from build123d import *

# Parameters (mm, degrees)
F2_ANGLE = 90
F0_W     = 20.32
F0_H     = 20.32
F3_DEPTH = 34.361461
F4_R     = 3.302
F5_DEPTH = 34.361461


with BuildPart() as f2:
    # F1 (on Right) → F2 (revolve)
    with BuildSketch(Plane.YZ):
        with BuildLine():
            ThreePointArc((44.45, -10.16), (34.29, 0), (44.45, 10.16))
            Line((44.45, 10.16), (44.45, 17.18023))
            Line((44.45, 17.18023), (0, 17.18023))
            Line((0, 17.18023), (0, 0))
            Line((0, 0), (0, -17.18023))
            Line((0, -17.18023), (44.45, -17.18023))
            Line((44.45, -17.18023), (44.45, -10.16))
        make_face()
    revolve(axis=Axis((0, 0, 26.599785), (0, 0, 1)), revolution_arc=F2_ANGLE)

    # F0 (on face) → F3 (cut, through all)
    with BuildSketch(Plane(origin=(0, 0, -17.18023), x_dir=(1, 0, 0), z_dir=(0, 0, -1))):
        with Locations((-10.16, -10.16)):
            Rectangle(F0_W, F0_H)
    extrude(amount=-F3_DEPTH, mode=Mode.SUBTRACT)

    # F4 (on face) → F5 (cut, through all)
    with BuildSketch(Plane(origin=(0, 0, -17.18023), x_dir=(1, 0, 0), z_dir=(0, 0, -1))):
        with Locations((-29.21, -7.62)):
            Circle(F4_R)
        with Locations((-7.62, -29.21)):
            Circle(F4_R)
    extrude(amount=-F5_DEPTH, mode=Mode.SUBTRACT)


solid = f2.part
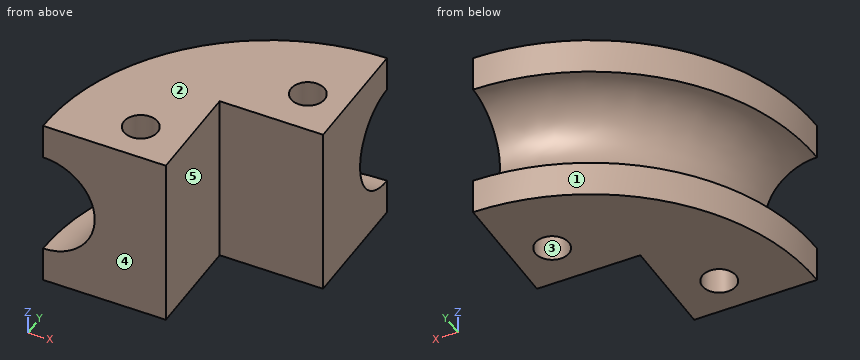
The model under review builds one solid part; all positions refer to its coordinate system, in mm. Face numbers are marked on the shaded views. A direction names the side the tool comes from. Coordinates: 2 decimals unless noted, no trailing zeros. Order: outer loops, then holes, each group sorted by start corner. A loop starts at its lowest first (then second) coordinate and runs counter-clockwise, first axis right, second up. Notation, with made-up numbers: (-12, -18) -> (35, -18) arc R20 cw to (35, -2) -> close; hole circle Ø2 at (77.5, -37). An arc over 180 degrees is marked (long way). Answer in a Markdown table with one row per item.
(1) Consider section A-A (z = -12). Write out the cut boundary in (x, y).
Answers:
| item | result |
|---|---|
| outline | (-44.45, 0) -> (-20.32, 0) -> (-20.32, 20.32) -> (0, 20.32) -> (0, 44.45) arc R44.45 ccw to start; hole circle Ø6.6 at (-29.21, 7.62); hole circle Ø6.6 at (-7.62, 29.21) |
(2) The part is to be moulded in two halves that separate along X. For the marked faces 1, 2 and 3, say which applies: +X half, -X half, draft (parallel to the pull), parting line (faces both ways), or undercut.
Answers:
| item | result |
|---|---|
| face 1 | -X half |
| face 2 | draft |
| face 3 | undercut |
(3) Insertion check: pin 1 (3 mm diameter, centred on x = -17, z = 12.5, fed in from -Y); pin 2 (10 mm diameter, centred on y = 13, z = -2, fed in from +X); pin 3 (6 mm diameter, centred on x = -7.62, y = 29.21, fed in from +Z). Each pin has a flat end and moves straight along its axis. Give the tip position at first contact, or say it passes through.
Answers:
| item | result |
|---|---|
| pin 1 | y = 20.32 |
| pin 2 | x = -20.32 |
| pin 3 | through |
(4) Wall thickness on line 1 along Y through (x, z) = (-28, -12); line 2 along X through (y, z) = (29, 7); line 3 along X through (y, z) = (29.21, -6.5): over which ranges is each line inside the solid? List them lowest first.
Answers:
| item | result |
|---|---|
| line 1 | 0 to 4.55, 10.69 to 34.52 |
| line 2 | -23.12 to -10.92, -4.32 to 0 |
| line 3 | -22.12 to -10.92, -4.32 to 0 |
(5) Consider section B-B (z = -4.5). Write out the cut boundary in (x, y), plus the area to 3 significant figures.
Answers:
| item | result |
|---|---|
| outline | (-35.34, 0) -> (-20.32, 0) -> (-20.32, 20.32) -> (0, 20.32) -> (0, 35.34) arc R35.34 ccw to start; hole circle Ø6.6 at (-29.21, 7.62); hole circle Ø6.6 at (-7.62, 29.21) |
| area | 500 mm² |
(6) Machinability: for the marked faces 4 and 5, which of the approach directions +Z, -Z, +X, -X, +Y, -Y give a long, thin tool a straight path to every point of the face, cutting with its end or side? Answer none if there is none.
Answers:
| item | result |
|---|---|
| face 4 | +Z, -Z, +X, -X, -Y |
| face 5 | +Z, -Z, +X, -Y |
